Could you check a few things on this drawing? It's one solid part, dimensions in mm from its lowest x, y, z. A direction names the side the tool comes from. Coordinates: 2 decimals unless noted, no trailing zeros. Order: outer loops, then holes, each group sorted by start corner. A loop starts at its lowest first (then second) coordinate and runs counter-clockwise, first axis right, second up. Notation, with made-up numbers: M 43.25,63.25 L 56.25,63.25 A21 cw 56.25,79.25 Z; hole C -30,-13.75 d4. An arc over 180 degrees is marked long. Answer as CSV lines item,"result". Start each with the question number.
1. I need wall thicknesses on line 1 along Z through (x, y) = (57.5, 30); line 2 along X through (y, z) = (63, 57.5); line 3 along Y through (x, z) = (82, 63.5). Which ranges of each line are inside material? Lowest first, please. Write a range as from..to.
2. If we section it at A-A (z = 58): List the corners of the cut face in (x, y) for me, plus the area to 3 significant figures.
3. If we section it at B-B (y = 10): List the corners of the cut face in (x, z) for me.
4. On a 3-axis mill with a long thin cutter (end or side, diameter ignored), from which of +Z, -Z, +X, -X, +Y, -Y can I reach the whole of each face in a straight line? I mean the marked faces 1, 2 and 3. Say none if no direction works.
5. Will these pins go through, and if not, where does the flat tip stop? pin 1 (5 mm diameter, centred on x = 17.5, z = 83.5, fed in from -Y); pin 2 (5 mm diameter, centred on y = 28.5, z = 41.5, fed in from +X) (3 decimals); pin 3 (6 mm diameter, centred on y = 31.5, z = 98, fed in from -X).
6. If we section it at C-C (y = 62): List the corners of the cut face in (x, z) for me.
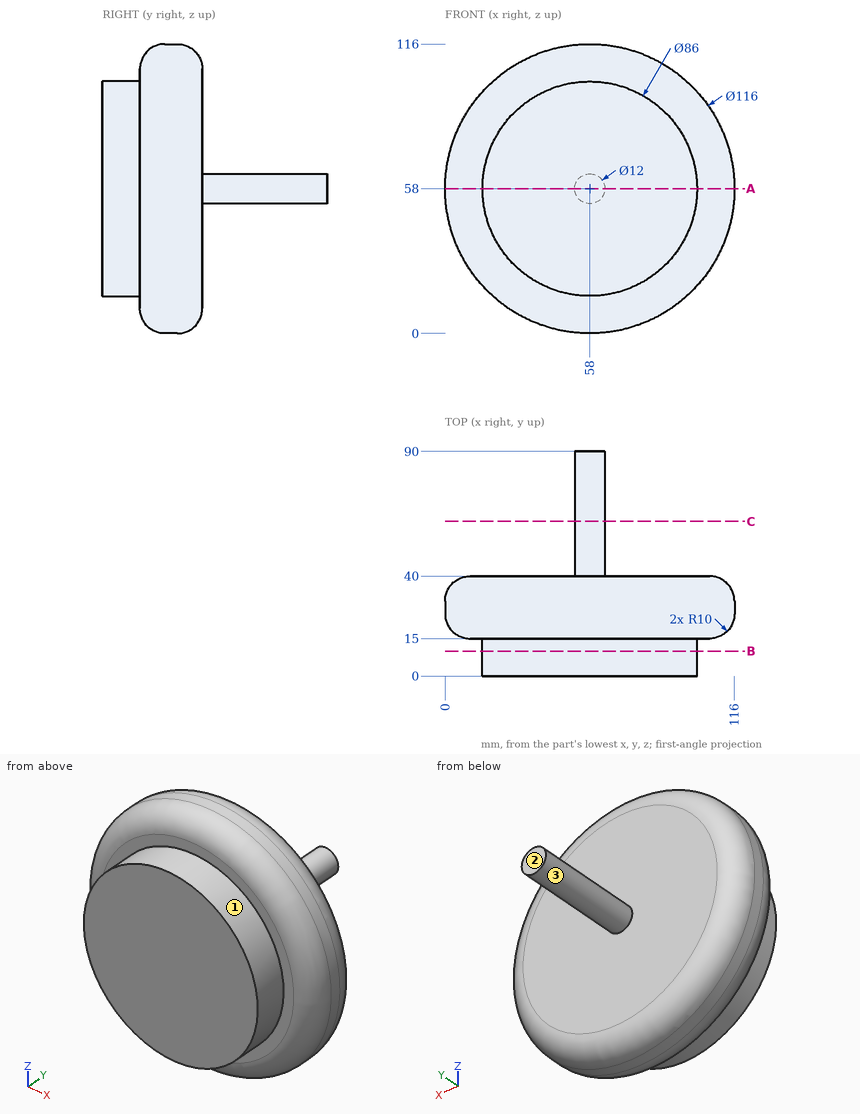
Solved:
1,line 1,"0..116"
1,line 2,"52.02..63.98"
1,line 3,"0..40"
2,outline,"M 0,25 A10 ccw 10,15 L 15,15 L 15,0 L 101,0 L 101,15 L 106,15 A10 ccw 116,25 L 116,30 A10 ccw 106,40 L 64,40 L 64,90 L 52,90 L 52,40 L 10,40 A10 ccw 0,30 Z"
2,area,"4,700 mm²"
3,outline,"C 58,58 d86"
4,face 1,"-Y"
4,face 2,"+Z, -Z, +X, -X, +Y"
4,face 3,"+Y"
5,pin 1,"y = 15"
5,pin 2,"x = 114.285"
5,pin 3,"x = 13.43"
6,outline,"C 58,58 d12"
